```python
from build123d import *

# Parameters (mm, degrees)
SKETCH_1_W          = 6
SKETCH_1_H          = 14
SKETCH_1_R          = 1.25
EXTRUDE_1_DEPTH     = 6
SKETCH_2_R          = 1.25
CUT_EXTRUDE_1_DEPTH = 7


with BuildPart() as part:
    # 草图1 → 凸台-拉伸1 (new body)
    with BuildSketch(Plane(origin=(0, 0, 0), x_dir=(0, 0, -1), z_dir=(1, 0, 0))):
        Rectangle(SKETCH_1_W, SKETCH_1_H)
        with Locations((0, 4)):
            Circle(SKETCH_1_R, mode=Mode.SUBTRACT)
        with Locations((0, -4)):
            Circle(SKETCH_1_R, mode=Mode.SUBTRACT)
    extrude(amount=EXTRUDE_1_DEPTH)

    # 草图2 → 切除-拉伸1 (cut, through all)
    with BuildSketch(Plane.XY.offset(3)):
        with Locations((3, 0)):
            Circle(SKETCH_2_R)
    extrude(amount=-CUT_EXTRUDE_1_DEPTH, mode=Mode.SUBTRACT)


solid = part.part
```
Part model, mm, in its own coordinate system. Coordinates: 2 decimals unless noted, no trailing zeros. Write each loop counter-clockwise with the first axis right and the second up, starting at its lowest first coordinate (ties: lowest second). Pieces come first, ordered by that corner, then holes.
Item 1: Slice it at B-B (z = 0). Write the cut outline in (x, y), and give its area (3 significant figures).
Item 2: Probe line 1 (Y direction, x = 2.5, z = 0.6); line 2 (Y direction, x = 4, z = 0.3); line 3 (Y direction, x = 2.5, z = 1.6). List the from-to ranges inside material, lowest first.
Item 3: Slice it at A-A (y = -0.75). Write the cut outline in (x, z).
Item 4: Slice it at D-D (z = 1.95). Write the cut outline in (x, y).
Item 5: Slice it at C-C (x = 2.2). Write the cut outline in (y, z), and give its area (3 significant figures).
Item 6: Mould opens along Y. For faces 1 (the face through (0, 0, 0)), 2 (the face through (3, 7, 0)), 3 (the face through (2.96, 2.78, 0.27)) say: released by +Y, released by -Y, zero draft, split by the parting line, or undercut.
Results found:
1. outline: (0, -7) - (6, -7) - (6, -5.25) - (0, -5.25) - close; (0, -2.75) - (6, -2.75) - (6, 2.75) - (0, 2.75) - close; (0, 5.25) - (6, 5.25) - (6, 7) - (0, 7) - close; hole circle Ø2.5 at (3, 0)
1. area: 49.1 mm2
2. line 1: y = -7 to -5.1, -2.9 to -1.15, 1.15 to 2.9, 5.1 to 7
2. line 2: y = -7 to -5.21, -2.79 to -0.75, 0.75 to 2.79, 5.21 to 7
2. line 3: y = -7 to -1.15, 1.15 to 7
3. outline: (0, -3) - (2, -3) - (2, 3) - (0, 3) - close; (4, -3) - (6, -3) - (6, 3) - (4, 3) - close
4. outline: (0, -7) - (6, -7) - (6, 7) - (0, 7) - close; hole circle Ø2.5 at (3, 0)
5. outline: (-7, -3) - (-0.96, -3) - (-0.96, 3) - (-7, 3) - close; (0.96, -3) - (7, -3) - (7, 3) - (0.96, 3) - close; hole circle Ø2.5 at (-4, 0); hole circle Ø2.5 at (4, 0)
5. area: 62.7 mm2
6. face 1: zero draft
6. face 2: released by +Y
6. face 3: undercut
